```python
from build123d import *

# Parameters (mm, degrees)
F0_R     = 44.893499
F1_DEPTH = 301.28476
F2_SIZE  = 12.7
F3_R     = 30.964692
F4_DEPTH = 254
F5_SIZE  = 12.7
F7_D     = 7.62


with BuildPart() as f1:
    # F0 (on Front) → F1 (new body)
    with BuildSketch(Plane.XZ):
        Circle(F0_R)
    extrude(amount=F1_DEPTH)

    # F2
    f2_edges = [f1.edges().sort_by_distance(p)[0] for p in [
        (44.893499, -150.64238, 0),
        (-44.893499, 0, 0),
        (-44.893499, -301.28476, 0),
    ]]
    chamfer(f2_edges, length=F2_SIZE)

    # F3 (on Right) → F4 (join)
    with BuildSketch(Plane.YZ):
        with Locations((-147.05956, 0)):
            Circle(F3_R)
    extrude(amount=-F4_DEPTH)

    # F5
    f5_edges = [f1.edges().sort_by_distance(p)[0] for p in [
        (-254, -178.024252, 0),
    ]]
    chamfer(f5_edges, length=F5_SIZE)

    # F7 (through all)
    with Locations(Plane(origin=(-254, 0, 0), x_dir=(0, -1, 0), z_dir=(-1, 0, 0))):
        with Locations((147.05956, 0)):
            Hole(F7_D / 2)


solid = f1.part
```
Input: part model. Units: mm. Frame: model coordinates. A direction names the side the tool comes from. Coordinates: 2 decimals unless noted, no trailing zeros. Loops run counter-clockwise (first coordinate to the right, second up) from the corner with the lowest first, then second, coordinate; pieces in that order, holes last. Notation, with made-up numbers: (20.5, 30.5) -> (29.5, 30.5) arc R25 cw to (29.5, 46.5) -> close; hole circle Ø9 at (4.25, 24.5). An arc over 180 degrees is marked (long way). Use a Markdown table: item, result.
1) Material intervals for line 1 along X through (y, z) = (-73.5, 0); line 2 along X through (y, z) = (-13.5, 13); line 3 along Z through (x, y) = (14, -128), sorted ascending. Write a range as from..to.
Results found:
| item | result |
|---|---|
| line 1 | x = -44.89..44.89 |
| line 2 | x = -42.97..42.97 |
| line 3 | z = -42.65..42.65 |
2) Contact query for flat-ended pins moving along their axis: pin 1 (12 mm diameter, centred on x = -120.5, z = -25.5, fed in from -Y); pin 2 (6 mm diameter, centred on y = -147.06, z = 0, fed in from +X); pin 3 (1.5 mm diameter, centred on x = -157, z = 4.5, fed in from -Y); pin 4 (4 mm diameter, centred on x = -212, y = -130, fed in from +Z). Output: stop coordinate, or through.
Results found:
| item | result |
|---|---|
| pin 1 | stops at y = -171.11 |
| pin 2 | passes through |
| pin 3 | stops at y = -177.8 |
| pin 4 | stops at z = 27.06 |
3) Cut plane B-B (y = -97). Return the cut outline in (x, z), then the cut area to 3 significant figures.
Results found:
| item | result |
|---|---|
| outline | circle Ø89.79 at (0, 0) |
| area | 6,330 mm2 |
4) Cut plane A-A (z = 0). Return the cut outline in (x, y).
Results found:
| item | result |
|---|---|
| outline | (-254, -165.32) -> (-241.3, -178.02) -> (-44.89, -178.02) -> (-44.89, -288.58) -> (-32.19, -301.28) -> (32.19, -301.28) -> (44.89, -288.58) -> (44.89, -150.87) -> (-254, -150.87) -> close; (-254, -143.25) -> (44.89, -143.25) -> (44.89, -12.7) -> (32.19, 0) -> (-32.19, 0) -> (-44.89, -12.7) -> (-44.89, -116.09) -> (-241.3, -116.09) -> (-254, -128.79) -> close |
5) Access query for faces 1 (the cylindrical face through (42.82, -148.71, 13.48)), 2 (the conical face through (-253.383, -165.923, 0.83)). Directions: +Z, -Z, +X, -X, +Y, -Y. A direction counts if a zero-diameter tool reaches every point of the face in a straight line with its end or side. Return the directions, or none.
Results found:
| item | result |
|---|---|
| face 1 | none |
| face 2 | -X |
6) Cut plane C-C (x = -221.5). Return the cut outline in (y, z).
Results found:
| item | result |
|---|---|
| outline | circle Ø61.93 at (-147.06, 0); hole circle Ø7.62 at (-147.06, 0) |
7) Pull-direction query (Z, two-part tool) for faces 3 (the cylindrical face through (-135.441, -177.994, 1.361)), 4 (the cylindrical face through (-102.46, -143.54, -1.46)), 5 (the flat face through (-254, -147, -4)); classes: released by +Z, released by -Z, zero draft, split by the parting line, or undercut.
Results found:
| item | result |
|---|---|
| face 3 | split by the parting line |
| face 4 | undercut |
| face 5 | zero draft |
